Geometry: final body of the model. Coordinates: model frame, mm. Face numbers are marked on the shaded views. Give positions to 0.01 mm unless a question says otherwise; leave off trailing zeros. Order: outer loops, then holes, each group sorted by start corner. A loop starts at its lowest first (then second) coordinate and runs counter-clockwise, first axis right, second up. Notation, with made-up numbers: (12, 88.25) -> (31, 88.25) arc R16 ccw to (31, 101.25) -> close; hole circle Ø9 at (41.5, 11). An arc over 180 degrees is marked (long way). Answer in a Markdown table with one row per item. Add a question column.
Q1. Pull-direction query (X, two-part tool) for the marked faces 1 and 2; classes: +X half, -X half, draft (parallel to the pull), parting line (faces both ways), or undercut.
Q2. Cut plane C-C on z = 0. Return the cut outline in (x, y).
Q3. Cut plane B-B on x = 0. Return the cut outline in (y, z).
Q4. Cut plane D-D on x = 30. Return the cut outline in (y, z), and give its area (3 significant figures).
Q5. Contact query for flat-ended pins moving along their axis: P1, Ø3, axis at x = -22, z = -7.5, coming from the -Y side; P2, Ø4, axis at x = -9.5, z = 4.5, coming from the +Y side; P3, Ø14.5, axis at x = 0, z = 0, coming from the +Y side; P4, Ø1.5, axis at x = -5, z = 0, coming from the +Y side. Output: stop coordinate, or through.
Q6. Cut plane A-A on y = 1.25. Return the cut outline in (x, z).
Q7. Line query: line 1 along Z through (x, y) = (30, 1.2); line 2 along Z through (x, y) = (28.5, 0.7); line 3 along Y through (x, z) = (10.5, 6.5). Output: solid intervals per line, ascending. Write a range as from..to.
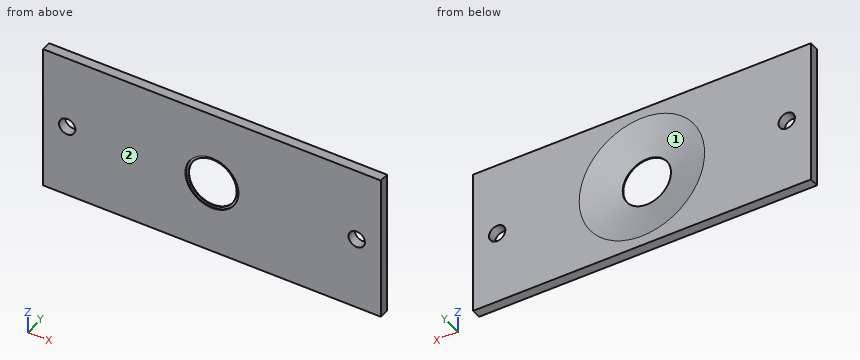
from build123d import *

# Parameters (mm, degrees)
SKETCH1_W            = 70
SKETCH1_H            = 30
SKETCH1_R            = 5
EXTRUDE1_DEPTH       = 2
CHAMFER1_SIZE        = 8
CHAMFER1_SIZE2       = 1.6
SKETCH3_R            = 5.5
CUT_EXTRUDE1_DEPTH   = 0.2
M3_CLEARANCE_HOLE1_D = 3.4


with BuildPart() as part:
    # Sketch1 → Extrude1 (new body)
    with BuildSketch(Plane(origin=(0, 0, 0), x_dir=(1, 0, 0), z_dir=(0, 1, 0))):
        Rectangle(SKETCH1_W, SKETCH1_H)
        Circle(SKETCH1_R, mode=Mode.SUBTRACT)
    extrude(amount=EXTRUDE1_DEPTH)

    # Chamfer1
    chamfer1_edges = [part.edges().sort_by_distance(p)[0] for p in [
        (-5, 2, 0),
    ]]
    chamfer1_side = [part.faces().sort_by_distance(p)[0] for p in [
        (0, 2, -14.238422689),
    ]]
    chamfer(chamfer1_edges, length=CHAMFER1_SIZE, length2=CHAMFER1_SIZE2, reference=chamfer1_side[0])

    # Sketch3 → Cut-Extrude1 (cut)
    with BuildSketch(Plane.XZ):
        Circle(SKETCH3_R)
    extrude(amount=-CUT_EXTRUDE1_DEPTH, mode=Mode.SUBTRACT)

    # M3 Clearance Hole1 (through all)
    with Locations(Plane(origin=(0, 2, 0), x_dir=(-1, 0, 0), z_dir=(0, 1, 0))):
        with Locations((-30, 0), (30, 0)):
            Hole(M3_CLEARANCE_HOLE1_D / 2)


solid = part.part
Completed:
| question | item | result |
|---|---|---|
| 1 | face 1 | undercut |
| 1 | face 2 | draft |
| 2 | outline | (-35, 0) -> (-31.7, 0) -> (-31.7, 2) -> (-35, 2) -> close; (-28.3, 0) -> (-5.5, 0) -> (-5.5, 0.2) -> (-5, 0.2) -> (-5, 0.4) -> (-13, 2) -> (-28.3, 2) -> close; (5, 0.2) -> (5.5, 0.2) -> (5.5, 0) -> (28.3, 0) -> (28.3, 2) -> (13, 2) -> (5, 0.4) -> close; (31.7, 0) -> (35, 0) -> (35, 2) -> (31.7, 2) -> close |
| 3 | outline | (0, -15) -> (2, -15) -> (2, -13) -> (0.4, -5) -> (0.2, -5) -> (0.2, -5.5) -> (0, -5.5) -> close; (0, 5.5) -> (0.2, 5.5) -> (0.2, 5) -> (0.4, 5) -> (2, 13) -> (2, 15) -> (0, 15) -> close |
| 4 | outline | (0, -15) -> (2, -15) -> (2, -1.7) -> (0, -1.7) -> close; (0, 1.7) -> (2, 1.7) -> (2, 15) -> (0, 15) -> close |
| 4 | area | 53.2 mm² |
| 5 | P1 | stops at y = 0 |
| 5 | P2 | stops at y = 1.9 |
| 5 | P3 | stops at y = 0.85 |
| 5 | P4 | stops at y = 0.55 |
| 6 | outline | (-35, -15) -> (35, -15) -> (35, 15) -> (-35, 15) -> close; hole circle Ø3.4 at (-30, 0); hole circle Ø18.5 at (0, 0); hole circle Ø3.4 at (30, 0) |
| 7 | line 1 | z = -15..-1.7, 1.7..15 |
| 7 | line 2 | z = -15..-0.8, 0.8..15 |
| 7 | line 3 | y = 0..1.87 |
